```python
from build123d import *

# Parameters (mm, degrees)
DISCO_START                  = 420
SK_DISCO_R                   = 55
DISCO_DEPTH                  = 6
PASANTES_M2_5_ROTOR_J4_START = 420
SK_PASANTES_M2_5_ROTOR_J4_R  = 1.45
PASANTES_M2_5_ROTOR_J4_DEPTH = 6
CAJAS_M2_5_START             = 423.5
SK_CAJAS_M2_5_R              = 2.75
CAJAS_M2_5_DEPTH             = 2.5
PASO_CABLE_START             = 420
SK_PASO_CABLE_R              = 3
PASO_CABLE_DEPTH             = 6
PASANTES_M4_ANGULOS_START    = 420
SK_PASANTES_M4_ANGULOS_R     = 2.25
PASANTES_M4_ANGULOS_DEPTH    = 6


with BuildPart() as part:
    # Sk_Disco → Disco (new body)
    with BuildSketch(Plane.XY.offset(DISCO_START)):
        Circle(SK_DISCO_R)
    extrude(amount=DISCO_DEPTH)

    # Sk_Pasantes_M2-5_rotor_J4 → Pasantes_M2-5_rotor_J4 (cut)
    with BuildSketch(Plane.XY.offset(PASANTES_M2_5_ROTOR_J4_START)):
        with Locations((12.390194253, -1.653204878)):
            Circle(SK_PASANTES_M2_5_ROTOR_J4_R)
        with Locations((7.626814549, 9.903620542)):
            Circle(SK_PASANTES_M2_5_ROTOR_J4_R)
        with Locations((-4.763379704, 11.55682542)):
            Circle(SK_PASANTES_M2_5_ROTOR_J4_R)
        with Locations((-12.390194253, 1.653204878)):
            Circle(SK_PASANTES_M2_5_ROTOR_J4_R)
        with Locations((-7.626814549, -9.903620542)):
            Circle(SK_PASANTES_M2_5_ROTOR_J4_R)
        with Locations((4.763379704, -11.55682542)):
            Circle(SK_PASANTES_M2_5_ROTOR_J4_R)
    extrude(amount=PASANTES_M2_5_ROTOR_J4_DEPTH, mode=Mode.SUBTRACT)

    # Sk_Cajas_M2-5 → Cajas_M2-5 (cut)
    with BuildSketch(Plane.XY.offset(CAJAS_M2_5_START)):
        with Locations((12.390194253, -1.653204878)):
            Circle(SK_CAJAS_M2_5_R)
        with Locations((7.626814549, 9.903620542)):
            Circle(SK_CAJAS_M2_5_R)
        with Locations((-4.763379704, 11.55682542)):
            Circle(SK_CAJAS_M2_5_R)
        with Locations((-12.390194253, 1.653204878)):
            Circle(SK_CAJAS_M2_5_R)
        with Locations((-7.626814549, -9.903620542)):
            Circle(SK_CAJAS_M2_5_R)
        with Locations((4.763379704, -11.55682542)):
            Circle(SK_CAJAS_M2_5_R)
    extrude(amount=CAJAS_M2_5_DEPTH, mode=Mode.SUBTRACT)

    # Sk_Paso_cable → Paso_cable (cut)
    with BuildSketch(Plane.XY.offset(PASO_CABLE_START)):
        Circle(SK_PASO_CABLE_R)
    extrude(amount=PASO_CABLE_DEPTH, mode=Mode.SUBTRACT)

    # Sk_Pasantes_M4_angulos → Pasantes_M4_angulos (cut)
    with BuildSketch(Plane.XY.offset(PASANTES_M4_ANGULOS_START)):
        with Locations((-10, -38.61)):
            Circle(SK_PASANTES_M4_ANGULOS_R)
        with Locations((-10, 38.61)):
            Circle(SK_PASANTES_M4_ANGULOS_R)
        with Locations((10, -38.61)):
            Circle(SK_PASANTES_M4_ANGULOS_R)
        with Locations((10, 38.61)):
            Circle(SK_PASANTES_M4_ANGULOS_R)
    extrude(amount=PASANTES_M4_ANGULOS_DEPTH, mode=Mode.SUBTRACT)


solid = part.part
```
The listing builds one solid part. Answer for the finished solid, in the listing's coordinates (mm). A direction names the side the tool comes from. Round coordinates to 2 decimals unless told otherwise and drop trailing zeros. Write each loop counter-clockwise with the first axis right and the second up, starting at its lowest first coordinate (ties: lowest second). Pieces come first, ordered by that corner, then holes. Notation, with made-up numbers: (26, 2.5) -> (78, 2.5) arc R27 ccw to (78, 18.5) -> close; hole circle Ø10 at (-36.5, -7.5). An arc over 180 degrees is marked (long way). Use CSV: the item, a comma, the result in double quotes. Start each with the question number.
(1) Section B-B on y = 38.61 is taken. Give the vertices of the cut face in (x, z), then the cut area to 3 significant figures.
(2) Each of these flat-tipped pins is pushed along its axis until it touches: pin 1 (3 mm diameter, centred on x = -12, y = 0.5, fed in from +Z); pin 2 (1.7 mm diameter, centred on x = 7.63, y = 9.9, fed in from +Z); pin 3 (1 mm diameter, centred on x = -19, z = 425, fed in from -Y); pin 4 (9 mm diameter, centred on x = 12.39, y = -1.65, fed in from +Z). Where does it stop, or does it pass through?
(3) Section A-A on x = 0 is taken. Give the vertices of the cut face in (y, z), then the cut area to 3 significant figures.
(4) Consider L1, parallel to Y at x = -12, z = 420.95; L2, parallel to Y at x = 13, z = 424.55; L3, parallel to X at y = -1.5, z = 420.4. Determine where each line is inside the solid, lowest interval first. Write a range as from..to.
(5) Which of the six approach directions +Z, -Z, +X, -X, +Y, -Y give full straight-line access (tool end or side, diameter ignored) to faces 3 (the face through (-5.121, 14.283, 424.732)), 4 (the face through (-6.244, -9.468, 421.726))?
(6) Section D-D on x = 32.5 is taken. Give the vertices of the cut face in (y, z), then the cut area to 3 significant figures.
(7) Section C-C on z = 421.25 is taken. Count the separate pieces of the cut face and the enclosed holes in it, then the cut area to 3 significant figures.
(8) The mould has two halves that part along X. Classify faces 1 (the face through (-1, -11, 420)), 2 (the face through (-6, -11, 423.5)): released by +X, released by -X, zero draft, split by the parting line, or undercut.
A:
1,outline,"(-39.17, 420) -> (-12.25, 420) -> (-12.25, 426) -> (-39.17, 426) -> close; (-7.75, 420) -> (7.75, 420) -> (7.75, 426) -> (-7.75, 426) -> close; (12.25, 420) -> (39.17, 420) -> (39.17, 426) -> (12.25, 426) -> close"
1,area,"416 mm²"
2,pin 1,"stops at z = 423.5"
2,pin 2,"passes through"
2,pin 3,"stops at y = -51.8"
2,pin 4,"stops at z = 426"
3,outline,"(-55, 420) -> (-3, 420) -> (-3, 426) -> (-55, 426) -> close; (3, 420) -> (55, 420) -> (55, 426) -> (3, 426) -> close"
3,area,"624 mm²"
4,L1,"y = -53.67..-39.64, -37.58..0.26, 3.05..37.58, 39.64..53.67"
4,L2,"y = -53.44..-4.33, 1.03..53.44"
4,L3,"x = -54.98..-2.6, 2.6..10.95, 13.83..54.98"
5,face 3,"+Z"
5,face 4,"+Z, -Z"
6,outline,"(-44.37, 420) -> (44.37, 420) -> (44.37, 426) -> (-44.37, 426) -> close"
6,area,"532 mm²"
7,separate pieces,"1"
7,enclosed holes,"11"
7,area,"9,370 mm²"
8,face 1,"zero draft"
8,face 2,"undercut"
